Read the model definition and answer for the solid it produces. Units are mm, in the model's axes. A direction names the side the tool comes from. Coordinates: 2 decimals unless noted, no trailing zeros. Write each loop counter-clockwise with the first axis right and the second up, starting at its lowest first coordinate (ties: lowest second). Pieces come first, ordered by that corner, then holes. Notation, with made-up numbers: (-36, 63) - (3, 63) arc R13 ccw to (3, 85) - close; hole circle Ø3 at (11, 18). An arc over 180 degrees is marked (long way). Return JSON: item names as keys, results as strings.
```python
from build123d import *

# Parameters (mm, degrees)
SKETCH1_R           = 12.4
BOSS_EXTRUDE1_DEPTH = 6.8
SKETCH2_R           = 5.8
BOSS_EXTRUDE2_DEPTH = 2
SKETCH3_R           = 3
CUT_EXTRUDE1_DEPTH  = 20.620397549
SKETCH4_R           = 2.05
CUT_EXTRUDE2_DEPTH  = 19.808508713
SKETCH5_R           = 2.05
CUT_EXTRUDE3_DEPTH  = 6


with BuildPart() as part:
    # Sketch1 → Boss-Extrude1 (new body)
    with BuildSketch(Plane.XY):
        Circle(SKETCH1_R)
    extrude(amount=BOSS_EXTRUDE1_DEPTH)

    # Sketch2 → Boss-Extrude2 (add)
    with BuildSketch(Plane.XY.offset(6.8)):
        Circle(SKETCH2_R)
    extrude(amount=BOSS_EXTRUDE2_DEPTH)

    # Sketch3 → Cut-Extrude1 (cut, through all)
    with BuildSketch(Plane.XY.offset(8.8)):
        Circle(SKETCH3_R)
    extrude(amount=-CUT_EXTRUDE1_DEPTH, mode=Mode.SUBTRACT)

    # Sketch4 → Cut-Extrude2 (cut, through all)
    with BuildSketch(Plane.XY.offset(6.8)):
        with Locations((4.35, 7.5)):
            Circle(SKETCH4_R)
        with Locations(Location((-4.35, 7.5, 0), (0, 0, 180))):
            Circle(SKETCH4_R)
        with Locations(Location((4.35, -7.5, 0), (0, 0, 180))):
            Circle(SKETCH4_R)
        with Locations((-4.35, -7.5)):
            Circle(SKETCH4_R)
    extrude(amount=-CUT_EXTRUDE2_DEPTH, mode=Mode.SUBTRACT)

    # Sketch5 → Cut-Extrude3 (cut)
    with BuildSketch(Plane(origin=(12.4, 0, 0), x_dir=(0, 0, -1), z_dir=(1, 0, 0))):
        with Locations((-3.271849547, 0)):
            Circle(SKETCH5_R)
    extrude(amount=-CUT_EXTRUDE3_DEPTH, mode=Mode.SUBTRACT)


solid = part.part
```
(1) Which of the six approach directions +Z, -Z, +X, -X, +Y, -Y give full straight-line access (tool end or side, diameter ignored) to faces 4 (the face through (6.4, 0, 3)), 5 (the face through (5.3, 2.9, 6.8)), 6 (the face through (-6.24, 8.29, 3.45))?
Answer:
{"face 4": "+X", "face 5": "+Z", "face 6": "+Z, -Z"}
(2) Determine the mould class of faces 1 (the face through (9.44, 1.39, 4.78)), 2 (the face through (-5.794, 0.255, 7.786)), 3 (the face through (2.5, -2.5, 8.8)) for opening direction Y: +Y half, -Y half, draft (parallel to the pull), parting line (faces both ways), or undercut.
Answer:
{"face 1": "undercut", "face 2": "parting line", "face 3": "draft"}
(3) Flat-ended cylindrical pins translate along their axes: P1, Ø3.5, axis at y = -1, z = 3.5, coming from the +X side; P2, Ø3.5, axis at y = 0, z = 3.27, coming from the +X side. Find the tip coordinate at first contact, or state that the pin passes through.
Answer:
{"P1": "x = 12.38", "P2": "x = 6.4"}
(4) A cutting plane is placed at D-D (y = 7.5). Determine the outline of the cut face in (x, z), and give its area (3 significant figures).
Answer:
{"outline": "(-9.87, 0) - (-6.4, 0) - (-6.4, 6.8) - (-9.87, 6.8) - close; (-2.3, 0) - (2.3, 0) - (2.3, 6.8) - (-2.3, 6.8) - close; (6.4, 0) - (9.87, 0) - (9.87, 6.8) - (6.4, 6.8) - close", "area": "78.5 mm²"}
(5) Straight lines are drawn through the part: line 1 (X direction, y = -9.25, z = 5); line 2 (Y direction, x = 4.35, z = 4.75); line 3 (Z direction, x = -7.25, y = -2.25). For each, find the intervals that lie inside material, in ascending order. Write a range as from..to.
Answer:
{"line 1": "-8.26..-5.42, -3.28..3.28, 5.42..8.26", "line 2": "-11.61..-9.55, -5.45..5.45, 9.55..11.61", "line 3": "0..6.8"}
(6) A cutting plane is placed at B-B (z = 5.75). Determine the outline of the cut face in (x, y).
Answer:
{"outline": "circle Ø24.8 at (0, 0); hole circle Ø4.1 at (-4.35, -7.5); hole circle Ø4.1 at (-4.35, 7.5); hole circle Ø6 at (0, 0); hole circle Ø4.1 at (4.35, -7.5); hole circle Ø4.1 at (4.35, 7.5)"}
(7) A cutting plane is placed at C-C (x = -4.35). Determine the outline of the cut face in (y, z).
Answer:
{"outline": "(-11.61, 0) - (-9.55, 0) - (-9.55, 6.8) - (-11.61, 6.8) - close; (-5.45, 0) - (5.45, 0) - (5.45, 6.8) - (3.84, 6.8) - (3.84, 8.8) - (-3.84, 8.8) - (-3.84, 6.8) - (-5.45, 6.8) - close; (9.55, 0) - (11.61, 0) - (11.61, 6.8) - (9.55, 6.8) - close"}
(8) A cutting plane is placed at A-A (y = 0). Determine the outline of the cut face in (x, z).
Answer:
{"outline": "(-12.4, 0) - (-3, 0) - (-3, 8.8) - (-5.8, 8.8) - (-5.8, 6.8) - (-12.4, 6.8) - close; (3, 0) - (12.4, 0) - (12.4, 1.22) - (6.4, 1.22) - (6.4, 5.32) - (12.4, 5.32) - (12.4, 6.8) - (5.8, 6.8) - (5.8, 8.8) - (3, 8.8) - close"}
